Check sheet for the drawn part. Datum: minimum x, y, z corner. Units: mm. Coordinates: 2 decimals unless noted, no trailing zeros. Order: outer loops, then holes, each group sorted by start corner. A loop starts at its lowest first (then second) coordinate and runs counter-clockwise, first axis right, second up.
Q1. Cross-section at D-D, the plane y = 0.5. Record the boundary of the cut face in (x, z).
Q2. Depth check by flat-ended pin: P1, Ø5, axis at x = 10.5, z = 11, coming from the -Y side; P2, Ø3, axis at x = 9, z = 11, coming from the -Y side (1 decimal). Enter the tip coordinate at first touch or a pass-through.
Q3. Cross-section at C-C, the plane y = 3.5. Record the boundary of the cut face in (x, z), and give its area (3 significant figures).
Q4. Draft check along Y on the marked faces 1, 2, 3 and 4. Enter one of: pulls with the +Y half, pulls with the -Y half, needs draft (parallel to the pull), parting line crosses it, or undercut.
Q5. Thickness scan on line 1 (Y direction, x = 11, z = 11.25) (1 decimal); line 2 (Z direction, x = 12.75, y = 2.5) (1 decimal); line 3 (Z direction, x = 9, y = 1.5) (1 decimal). Record the ranges inside material, lowest first.
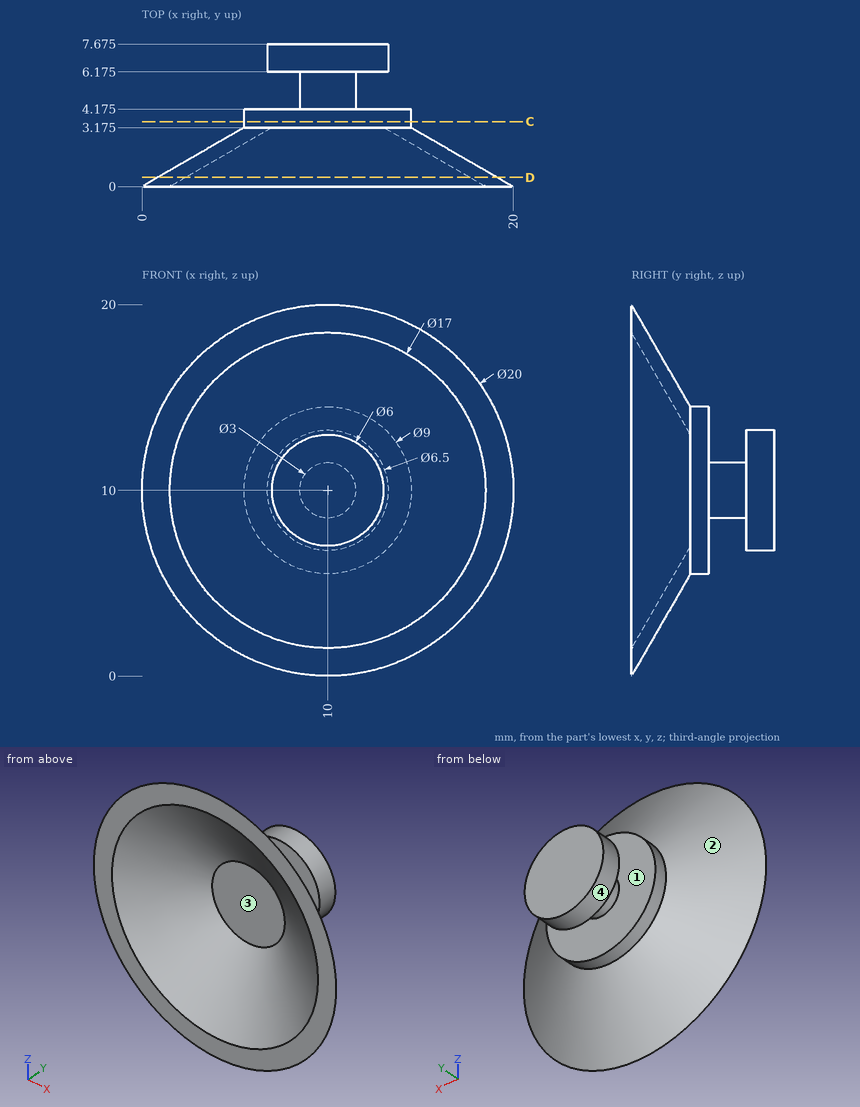
Check values:
1. outline: circle Ø18.27 at (10, 10); hole circle Ø15.27 at (10, 10)
2. P1: stops at y = 2.82
2. P2: stops at y = 3.2
3. outline: circle Ø9 at (10, 10)
3. area: 63.6 mm2
4. face 1: undercut
4. face 2: pulls with the +Y half
4. face 3: pulls with the -Y half
4. face 4: needs draft
5. line 1: y = 3.2 to 4.2, 6.2 to 7.7
5. line 2: z = 5 to 6.9, 13.1 to 15
5. line 3: z = 2.7 to 4.2, 15.8 to 17.3
